from build123d import *

# Parameters (mm, degrees)
SKETCH1_R           = 50
BOSS_EXTRUDE1_DEPTH = 30
SKETCH2_R           = 50
BOSS_EXTRUDE2_DEPTH = 4
SKETCH3_W           = 11.6
SKETCH3_H           = 22.75
CUT_EXTRUDE1_DEPTH  = 14
SKETCH5_R           = 1.75
CUT_EXTRUDE3_DEPTH  = 79.460180984


with BuildPart() as part:
    # Sketch1 → Boss-Extrude1 (new body)
    with BuildSketch(Plane(origin=(0, 0, 0), x_dir=(1, 0, 0), z_dir=(0, 1, 0))):
        with Locations(Location((0, 0, 0), (0, 0, 270))):
            Circle(SKETCH1_R)
    extrude(amount=BOSS_EXTRUDE1_DEPTH)

    # Sketch2 → Boss-Extrude2 (add)
    with BuildSketch(Plane(origin=(0, 30, 0), x_dir=(1, 0, 0), z_dir=(0, 1, 0))):
        with Locations(Location((0, 0, 0), (0, 0, 270))):
            Circle(SKETCH2_R)
    extrude(amount=BOSS_EXTRUDE2_DEPTH)

    # Sketch3 → Cut-Extrude1 (cut)
    with BuildSketch(Plane(origin=(0, 34, 0), x_dir=(1, 0, 0), z_dir=(0, 1, 0))):
        with Locations((0, -6.375)):
            Rectangle(SKETCH3_W, SKETCH3_H)
    extrude(amount=-CUT_EXTRUDE1_DEPTH, mode=Mode.SUBTRACT)

    # Sketch5 → Cut-Extrude3 (cut, through all)
    with BuildSketch(Plane(origin=(0, 34, 0), x_dir=(1, 0, 0), z_dir=(0, 1, 0))):
        with Locations(Location((0, 40, 0), (0, 0, 270))):
            Circle(SKETCH5_R)
        with Locations(Location((40, 0, 0), (0, 0, 270))):
            Circle(SKETCH5_R)
        with Locations(Location((0, -40, 0), (0, 0, 270))):
            Circle(SKETCH5_R)
        with Locations(Location((-40, 0, 0), (0, 0, 270))):
            Circle(SKETCH5_R)
    extrude(amount=-CUT_EXTRUDE3_DEPTH, mode=Mode.SUBTRACT)


solid = part.part
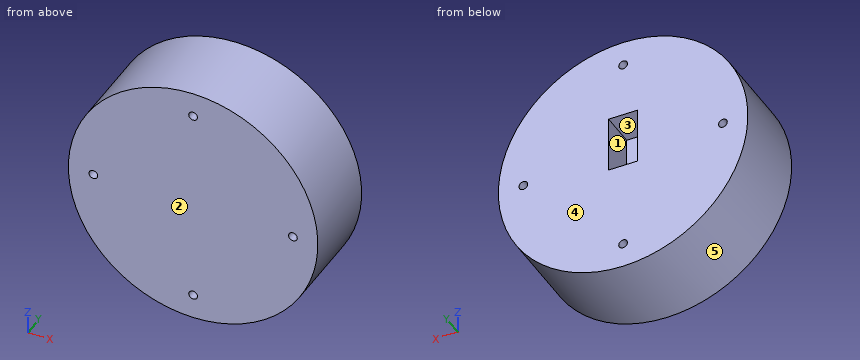
Can you work these out from the model? Positions are in its coordinate system, mm. Face numbers are marked on the shaded views. A direction names the side the tool comes from. Coordinates: 2 decimals unless noted, no trailing zeros. Loops run counter-clockwise (first coordinate to the right, second up) from the corner with the lowest first, then second, coordinate; pieces in that order, holes last. Notation, with made-up numbers: M -20.75,71.25 L 19.25,71.25 A10 cw 19.25,85.25 Z; hole C -7,-37.5 d7. An arc over 180 degrees is marked long. Return JSON: item names as keys, results as strings. Group by question number.
Item 1: If I drill on L1, parallel to X at y = 7, z = 0; L2, parallel to X at y = 21.5, z = 0; L3, parallel to Z at x = -1, y = 27, over which ranges is the centre line in solid material (lowest first)? Write a range as from..to.
Item 2: Imagine slicing it at D-D (x = 0). Please give me the cut outline in (y, z), and give its area (3 significant figures).
Item 3: I'm going to push flat-ended pins straight in: pin 1 Ø1 at (y, z) = (26, -28.5) entering from -X; pin 2 Ø8 at (y, z) = (17.5, 20.5) entering from +X; pin 3 Ø3.5 at (x, y) = (2, 24.5) entering from +Z. Where does each tip first touch, or does it pass through?
Item 4: Imagine slicing it at B-B (z = -40). Please give me the cut outline in (x, y).
Item 5: Thinking about a two-plate mould opening in X: for the marked faces 3, 4 and 5, which applies, released by +X, released by -X, zero draft, split by the parting line, or undercut?
Item 6: Imagine slicing it at A-A (x = -40). Please give me the cut outline in (y, z).
Item 7: Imagine slicing it at C-C (y = 29.5). Please give me the cut outline in (x, z), and give its area (3 significant figures).
Item 8: On a 3-axis mill with a long thin cutter (end or side, diameter ignored), from which of +Z, -Z, +X, -X, +Y, -Y can I reach the whole of each face in a straight line? I mean the marked faces 1 and 2. Say none if no direction works.
Verdict:
{
 "1": {"L1": "x = -50..-41.75, -38.25..38.25, 41.75..50", "L2": "x = -50..-41.75, -38.25..-5.8, 5.8..38.25, 41.75..50", "L3": "z = -49.99..-41.44, -38.56..-5, 17.75..38.56, 41.44..49.99"},
 "2": {"outline": "M 0,-50 L 34,-50 L 34,-41.75 L 0,-41.75 Z; M 0,-38.25 L 34,-38.25 L 34,-5 L 20,-5 L 20,17.75 L 34,17.75 L 34,38.25 L 0,38.25 Z; M 0,41.75 L 34,41.75 L 34,50 L 0,50 Z", "area": "2,840 mm^2"},
 "3": {"pin 1": "stops at x = -41.42", "pin 2": "stops at x = 47.2", "pin 3": "stops at z = 50"},
 "4": {"outline": "M -30,0 L -1.75,0 L -1.75,34 L -30,34 Z; M 1.75,0 L 30,0 L 30,34 L 1.75,34 Z"},
 "5": {"face 3": "undercut", "face 4": "zero draft", "face 5": "split by the parting line"},
 "6": {"outline": "M 0,-30 L 34,-30 L 34,-1.75 L 0,-1.75 Z; M 0,1.75 L 34,1.75 L 34,30 L 0,30 Z"},
 "7": {"outline": "C 0,0 d100; hole C -40,0 d3.5; hole M -5.8,-5 L 5.8,-5 L 5.8,17.75 L -5.8,17.75 Z; hole C 0,-40 d3.5; hole C 0,40 d3.5; hole C 40,0 d3.5", "area": "7,550 mm^2"},
 "8": {"face 1": "+Y", "face 2": "+Z, -Z, +X, -X, -Y"}
}
